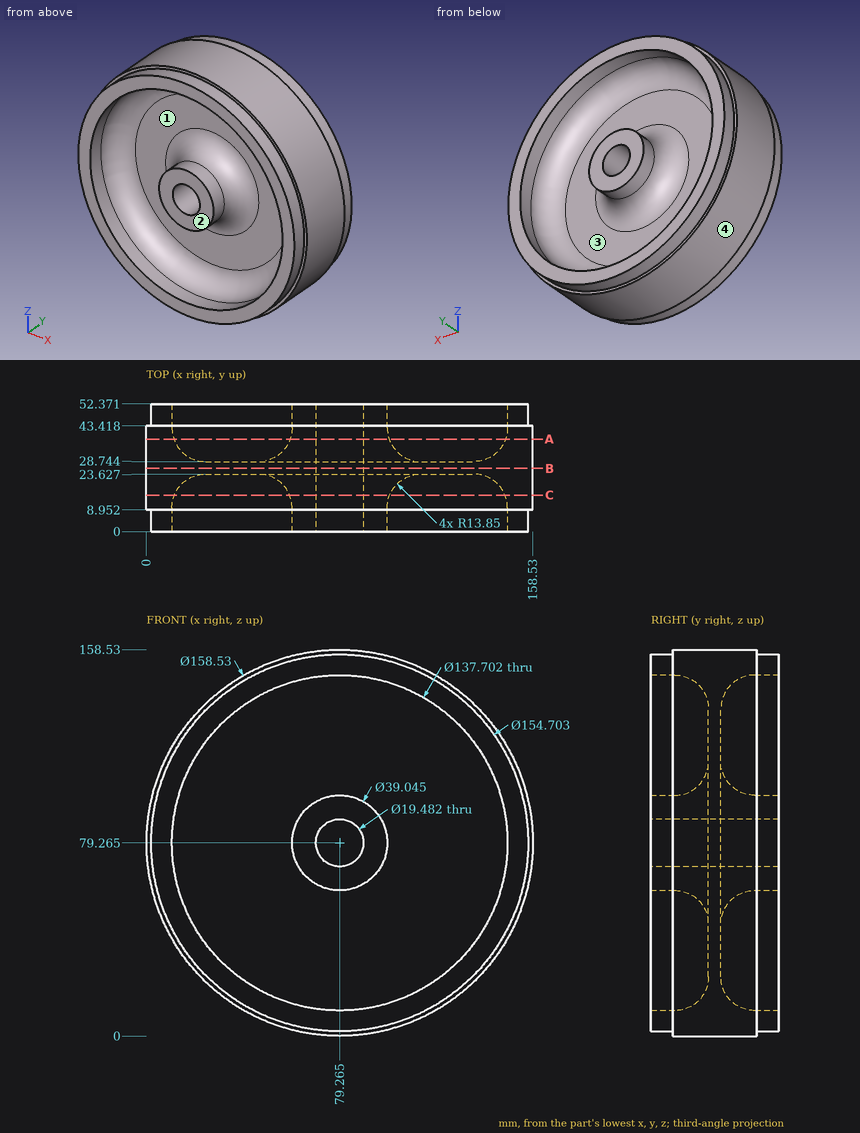
Source: three-view drawing plus pictorial views. Frame: mm from the lowest corner of the part. Give positions to 0.01 mm unless a question says otherwise; leave off trailing zeros. Loops run counter-clockwise (first coordinate to the right, second up) from the corner with the lowest first, then second, coordinate; pieces in that order, holes last. Notation, with made-up numbers: (86, -9) -> (137, -9) arc R37 cw to (137, 28) -> close; hole circle Ø7 at (16.25, 16.5). An arc over 180 degrees is marked (long way). Put each result on its own line as item: value. Start each with the question number.
1) Cut plane A-A (y = 38). Return loops of the section in (x, z) (1 decimal).
2) Draft query along Z for the marked faces 1, 2, 3 and 4. Return one class per face: released by +Z, released by -Z, zero draft, split by the parting line, or undercut.
3) Cut plane B-B (y = 26). Return loops of the section in (x, z) (1 decimal).
4) Contact query for flat-ended pins moving along their axis: P1, Ø2, axis at x = 93, z = 138, coming from the -Y side; P2, Ø4, axis at x = 40, y = 47, coming from the -Z side; P3, Ø10, axis at y = 38.5, z = 20, coming from the +X side; P4, Ø12, axis at x = 77.5, y = 13, coming from the +Z side. Output: stop coordinate, or through.
5) Cut plane C-C (y = 15). Return loops of the section in (x, z) (1 decimal), then the cut area to 3 significant figures.
6) Material intervals for probe 1 along Z at (x, y) = (66, 32) (1 decimal); probe 2 along X at (y, z) = (37, 65.5) (1 decimal); probe 3 along X at (y, z) = (6, 69) (1 decimal), sorted ascending.
Results are:
1. outline: circle Ø158.5 at (79.3, 79.3); circle Ø40.6 at (79.3, 79.3); hole circle Ø136.1 at (79.3, 79.3); hole circle Ø19.5 at (79.3, 79.3)
2. face 1: undercut
2. face 2: zero draft
2. face 3: undercut
2. face 4: split by the parting line
3. outline: circle Ø158.5 at (79.3, 79.3); hole circle Ø19.5 at (79.3, 79.3)
4. P1: stops at y = 22.1
4. P2: stops at z = 11.48
4. P3: stops at x = 137.04
4. P4: stops at z = 158.53
5. outline: circle Ø158.5 at (79.3, 79.3); circle Ø41.1 at (79.3, 79.3); hole circle Ø135.7 at (79.3, 79.3); hole circle Ø19.5 at (79.3, 79.3)
5. area: 6,310 mm2
6. probe 1: z = 1.1 to 16.7, 58.7 to 99.8, 141.8 to 157.4
6. probe 2: x = 1.2 to 13, 63.8 to 94.7, 145.5 to 157.3
6. probe 3: x = 2.6 to 11.2, 62.7 to 95.9, 147.3 to 155.9
